Work out the finished part from the listing and answer in its coordinate system (mm). A direction names the side the tool comes from. Give positions to 0.01 mm unless a question says otherwise; leave off trailing zeros. Order: outer loops, then holes, each group sorted by start corner. A loop starts at its lowest first (then second) coordinate and runs counter-clockwise, first axis right, second up. Notation, with made-up numbers: (49.5, -19) - (87.5, -19) arc R9 ccw to (87.5, -2) - close; hole circle Ø7 at (20, 62.5). An arc over 180 degrees is marked (long way). Write each question's results on one line, items separated by ' | '.
from build123d import *

# Parameters (mm, degrees)
BOSS_EXTRUDE3_DEPTH         = 28
SKETCH4_W                   = 32
SKETCH4_H                   = 74
CUT_EXTRUDE2_DEPTH          = 26
M6_TAPPED_HOLE1_D           = 5
M6_TAPPED_HOLE1_DEPTH       = 27
M6_TAPPED_HOLE1_CSINK_D     = 6
M6_TAPPED_HOLE1_CSINK_ANGLE = 90
M6_TAPPED_HOLE1_TIP         = 1.502151548
CHAMFER1_SIZE               = 2
FILLET2_R                   = 2


with BuildPart() as part:
    # Sketch3 → Boss-Extrude3 (new body, symmetric)
    with BuildSketch(Plane.XY):
        Polygon((12.5, 0), (-12.5, 0), (-12.5, 45), (-7.5, 84), (7.5, 84), (12.5, 45), align=None)
    extrude(amount=BOSS_EXTRUDE3_DEPTH, both=True)

    # Sketch4 → Cut-Extrude2 (cut, through all)
    with BuildSketch(Plane(origin=(12.5, 0, 0), x_dir=(0, 0, -1), z_dir=(1, 0, 0))):
        with Locations((0, 47)):
            Rectangle(SKETCH4_W, SKETCH4_H)
    extrude(amount=-CUT_EXTRUDE2_DEPTH, mode=Mode.SUBTRACT)

    # Sketch7 → CBORE for M4 Hex Socket Head Cap Screw1 (revolve, cut)
    with BuildSketch(Plane(origin=(0, 75, 28), x_dir=(0, -1, 0), z_dir=(1, 0, 0))):
        Polygon((0, 0), (0, 23.004303095), (5, 20), (5, 4.025), (5.025, 4), (6, 4), (6, 0), align=None)
    cbore_for_m4_hex_socket_head_cap_screw1 = revolve(axis=Axis((0, 75, 34.35), (0, 0, -1)), mode=Mode.SUBTRACT)

    # Mirror1: CBORE for M4 Hex Socket Head Cap Screw1 across plane
    add(cbore_for_m4_hex_socket_head_cap_screw1.mirror(Plane.XY), mode=Mode.SUBTRACT)

    # M6 Tapped Hole1
    with Locations(Plane.XY.offset(28)):
        with Locations((0, 20)):
            CounterSinkHole(M6_TAPPED_HOLE1_D / 2, M6_TAPPED_HOLE1_CSINK_D / 2, depth=M6_TAPPED_HOLE1_DEPTH, counter_sink_angle=M6_TAPPED_HOLE1_CSINK_ANGLE)
            with Locations((0, 0, -(M6_TAPPED_HOLE1_DEPTH + M6_TAPPED_HOLE1_TIP / 2))):  # 118° drill point
                Cone(0, M6_TAPPED_HOLE1_D / 2, M6_TAPPED_HOLE1_TIP, mode=Mode.SUBTRACT)

    # Chamfer1
    chamfer1_edges = [part.edges().sort_by_distance(p)[0] for p in [
        (12.5, 10, 0),
        (-12.5, 10, 0),
    ]]
    chamfer(chamfer1_edges, length=CHAMFER1_SIZE)

    # Fillet2
    fillet2_edges = [part.edges().sort_by_distance(p)[0] for p in [
        (-7.5, 84, 22),
        (7.5, 84, 22),
        (-7.5, 84, -22),
        (7.5, 84, -22),
    ]]
    fillet(fillet2_edges, radius=FILLET2_R)


solid = part.part
1. Straight lines are drawn through the part: line 1 (Y direction, x = 0, z = 19.5); line 2 (Y direction, x = 0, z = 25.35); line 3 (Z direction, x = 11.5, y = 27.5). For each, find the intervals that lie inside material, in ascending order. Write a range as [from, to].
Answer list:
line 1: [0, 17.5], [22.5, 70], [80, 84] | line 2: [0, 17.5], [22.5, 69], [81, 84] | line 3: [-28, -16], [16, 28]
2. A tool of negligible diameter and unlimited length cuts with its end or side. For faces 1 (the face through (11.5, 9, 0.2)), 2 (the face through (0, 81, -26)), 3 (the face through (0, 10, 0)), 4 (the face through (0, 81, 26)), from which of +Z, -Z, +X, -X, +Y, -Y can it reach the whole face along a straight path? Write none if from no direction.
Answer list:
face 1: +X, +Y | face 2: -Z | face 3: +X, -X, +Y | face 4: +Z
3. Given P1, Ø6.5, axis at x = 2, z = -5.5, coming from the +Y side; P2, Ø4, axis at y = 31, z = -12.5, coming from the -X side; P3, Ø9.5, axis at x = 0.5, y = 76, coming from the +Z side; P4, Ø6, axis at y = 49.5, z = 15, coming from the +X side, each flat-ended and moving along its own axis, determine where each tip first touches the part or whether it passes through.
Answer list:
P1: y = 10 | P2: through | P3: z = 24 | P4: x = 12.29
4. Determine the mould class of faces 5 (the face through (-7.05, 83.51, 21.92)), 6 (the face through (1.915, 70.381, 20.043)), 7 (the face through (0, 0, 0)), 8 (the face through (12.5, 7.8, 0.4)) for opening direction Y: +Y half, -Y half, draft (parallel to the pull), parting line (faces both ways), or undercut.
Answer list:
face 5: +Y half | face 6: undercut | face 7: -Y half | face 8: draft
5. A cutting plane is placed at C-C, the plane y = 75. Write down the section's boundary in (x, z) (3 decimals), then the cut area to 3 significant figures.
Answer list:
outline: (-8.654, -28) - (-6, -28) - (-6, -24) - (-5.025, -24) - (-5, -23.975) - (-5, -16) - (-8.654, -16) - close; (-8.654, 16) - (-5, 16) - (-5, 23.975) - (-5.025, 24) - (-6, 24) - (-6, 28) - (-8.654, 28) - close; (5, -23.975) - (5.025, -24) - (6, -24) - (6, -28) - (8.654, -28) - (8.654, -16) - (5, -16) - close; (5, 16) - (8.654, 16) - (8.654, 28) - (6, 28) - (6, 24) - (5.025, 24) - (5, 23.975) - close | area: 159 mm^2
6. A cutting plane is placed at D-D, the plane y = 51. Write down the section's boundary in (x, z).
Answer list:
outline: (-11.73, -28) - (11.73, -28) - (11.73, -16) - (-11.73, -16) - close; (-11.73, 16) - (11.73, 16) - (11.73, 28) - (-11.73, 28) - close
7. A cutting plane is placed at B-B, the plane y = 20. Write down the section's boundary in (x, z), then the cut area to 3 significant figures.
Answer list:
outline: (-12.5, -28) - (12.5, -28) - (12.5, -16) - (-12.5, -16) - close; (-12.5, 16) - (-2.5, 16) - (-2.5, 27.5) - (-3, 28) - (-12.5, 28) - close; (2.5, 16) - (12.5, 16) - (12.5, 28) - (3, 28) - (2.5, 27.5) - close | area: 540 mm^2
8. A cutting plane is placed at A-A, the plane z = 21. Write down the section's boundary in (x, y), then the cut area to 3 significant figures.
Answer list:
outline: (-12.5, 0) - (12.5, 0) - (12.5, 45) - (7.72, 82.25) arc R2 ccw to (5.74, 84) - (-5.74, 84) arc R2 ccw to (-7.72, 82.25) - (-12.5, 45) - close; hole circle Ø10 at (0, 75); hole circle Ø5 at (0, 20) | area: 1,810 mm^2
